```python
from build123d import *

# Parameters (mm, degrees)
BOSS_EXTRUDE1_DEPTH     = 12
SKETCH2_R               = 4
CUT_EXTRUDE1_DEPTH      = 46.675485921
SKETCH3_R               = 1
CUT_EXTRUDE2_DEPTH      = 46.67548588
FILLET2_R               = 1
SKETCH5_R               = 6
CUT_EXTRUDE3_DEPTH      = 10
CUT_EXTRUDE4_DEPTH      = 1
CUT_EXTRUDE4_DEPTH_BACK = 2


with BuildPart() as part:
    # Sketch1 → Boss-Extrude1 (new body)
    with BuildSketch(Plane.XY):
        with BuildLine():
            Line((0, 5), (0, 0))
            Line((0, 0), (20, 0))
            add(Edge.make_bspline(
                [(20, 0), (28.689683173, 0), (29.340198242, 2), (38, 2)],
                knots=[0, 0, 0, 0, 1, 1, 1, 1], degree=3))
            Line((38, 2), (40, 2))
            Line((40, 2), (40, 7))
            Line((40, 7), (34, 7))
            Line((34, 7), (34, 18.5))
            Line((34, 18.5), (28, 18.5))
            Line((28, 18.5), (28, 6.519175256))
            add(Edge.make_bspline(
                [(17, 5), (22.481298088, 5), (24.633063977, 5.927411475), (28, 6.519175256)],
                knots=[0, 0, 0, 0, 0.680959424, 0.680959424, 0.680959424, 0.680959424], degree=3))
            Line((17, 5), (0, 5))
        make_face()
    extrude(amount=BOSS_EXTRUDE1_DEPTH)

    # Sketch2 → Cut-Extrude1 (cut, through all)
    with BuildSketch(Plane(origin=(0, 0, 0), x_dir=(0, 0, -1), z_dir=(1, 0, 0))):
        with BuildLine():
            Line((0, 12.5), (0, 18.5))
            Line((0, 18.5), (-6, 18.5))
            ThreePointArc((-6, 18.5), (-1.757359313, 16.742640687), (0, 12.5))
        make_face()
        with BuildLine():
            ThreePointArc((-12, 12.5), (-10.242640687, 16.742640687), (-6, 18.5))
            Line((-6, 18.5), (-12, 18.5))
            Line((-12, 18.5), (-12, 12.5))
        make_face()
        with Locations(Location((-6, 12.5, 0), (0, 0, 180))):
            Circle(SKETCH2_R)
    extrude(amount=CUT_EXTRUDE1_DEPTH, mode=Mode.SUBTRACT)

    # Sketch3 → Cut-Extrude2 (cut, through all)
    with BuildSketch(Plane(origin=(0, 0, 0), x_dir=(1, 0, 0), z_dir=(0, 1, 0))):
        with Locations(Location((15, -6, 0), (0, 0, 270))):
            Circle(SKETCH3_R)
        with Locations(Location((5, -6, 0), (0, 0, 270))):
            Circle(SKETCH3_R)
    extrude(amount=CUT_EXTRUDE2_DEPTH, mode=Mode.SUBTRACT)

    # Fillet2
    fillet2_edges = [part.edges().sort_by_distance(p)[0] for p in [
        (0, 2.5, 12),
        (40, 4.5, 0),
        (0, 2.5, 0),
        (40, 4.5, 12),
    ]]
    fillet(fillet2_edges, radius=FILLET2_R)

    # Sketch5 → Cut-Extrude3 (cut)
    with BuildSketch(Plane(origin=(34, 0, 0), x_dir=(0, 0, -1), z_dir=(1, 0, 0))):
        with Locations((-6, 12.5)):
            Circle(SKETCH5_R)
    extrude(amount=CUT_EXTRUDE3_DEPTH, mode=Mode.SUBTRACT)

    # Sketch6 → Cut-Extrude4 (cut, two sides: drawn at the far end of the back side and taken through both)
    with BuildSketch(Plane(origin=(0, 5, 0), x_dir=(1, 0, 0), z_dir=(0, 1, 0)).offset(-CUT_EXTRUDE4_DEPTH_BACK)):
        Polygon((12.85, -4.758696921), (12.85, -7.241303079), (15, -8.482606158), (17.15, -7.241303079), (17.15, -4.758696921), (15, -3.517393842), align=None)
        Polygon((5, -3.517393842), (2.85, -4.758696921), (2.85, -7.241303079), (5, -8.482606158), (7.15, -7.241303079), (7.15, -4.758696921), align=None)
    extrude(amount=CUT_EXTRUDE4_DEPTH + CUT_EXTRUDE4_DEPTH_BACK, mode=Mode.SUBTRACT)


solid = part.part
```
The model under review builds one solid part; all positions refer to its coordinate system, in mm. A direction names the side the tool comes from. Round coordinates to 2 decimals unless told otherwise and drop trailing zeros. Loops run counter-clockwise (first coordinate to the right, second up) from the corner with the lowest first, then second, coordinate; pieces in that order, holes last. Notation, with made-up numbers: (-8, 14.25) - (4, 14.25) arc R22 cw to (4, 26.25) - close; hole circle Ø4 at (89, 5). An arc over 180 degrees is marked (long way). Use a Markdown table: item, result. Add a question column.
Q1. Machinability: for faces 5 (the face through (9, 5, 6)), 6 (the face through (13.94, 3.99, 4.13)), 7 (the face through (37, 7, 2)), which of the approach directions +Z, -Z, +X, -X, +Y, -Y give a long, thin tool a straight path to every point of the face, cutting with its end or side? Answer none if there is none.
Q2. For probe 1 along Z at (x, y) = (15, 2.1); probe 2 along Z at (x, y) = (32, 12.25); probe 3 along X at (y, z) = (3.75, 4), list the stretches that pass through material, from the lowest coordinate up.
Q3. Insertion check: pin 1 Ø6 at (x, z) = (24.5, 9.5) entering from -Y; pin 2 Ø3.5 at (y, z) = (10, 7) entering from +X; pin 3 Ø1.8 at (x, z) = (38, 1.5) entering from +Y; pin 4 Ø1.8 at (x, z) = (15, 6) entering from -Y. Each pin has a flat end and moves straight along its axis. Give the tip position at first contact, or say it passes through.
Q4. The part is to be moulded in two halves that separate along Z. For faces 1 (the face through (19.7, 4.9, 0)), 2 (the face through (39, 2, 6)), 3 (the face through (39.699, 4.535, 11.715)), 4 (the face through (2.85, 4, 6)), say which applies: pulls with the +Z half, pulls with the -Z half, needs draft (parallel to the pull), parting line crosses it, or undercut.
Q5. Add section A-A (y = 9.5). State the section outline as (x, z) points.
Q6. Add section B-B (x = 16.5). State the section outline as (y, z) points.
Worked answers:
| question | item | result |
|---|---|---|
| 1 | face 5 | +Z, -Z, -X, +Y |
| 1 | face 6 | +Y |
| 1 | face 7 | +Z, -Z, +X, +Y |
| 2 | probe 1 | 0 to 5, 7 to 12 |
| 2 | probe 2 | 0 to 2.01, 9.99 to 12 |
| 2 | probe 3 | 0 to 4.16, 5.84 to 14.16, 15.84 to 40 |
| 3 | pin 1 | y = 0.02 |
| 3 | pin 2 | x = 34 |
| 3 | pin 3 | y = 7 |
| 3 | pin 4 | through |
| 4 | face 1 | pulls with the -Z half |
| 4 | face 2 | needs draft |
| 4 | face 3 | pulls with the +Z half |
| 4 | face 4 | undercut |
| 5 | outline | (28, 0) - (34, 0) - (34, 3.35) - (28, 3.35) - close; (28, 8.65) - (34, 8.65) - (34, 12) - (28, 12) - close |
| 6 | outline | (0, 0) - (5, 0) - (5, 4.38) - (3, 4.38) - (3, 7.62) - (5, 7.62) - (5, 12) - (0, 12) - close |
